Check sheet for the modelled part. Datum: model origin and axes. Units: mm. A direction names the side the tool comes from. Coordinates: 2 decimals unless noted, no trailing zeros. Write each loop counter-clockwise with the first axis right and the second up, starting at its lowest first coordinate (ties: lowest second). Pieces come first, ordered by that corner, then holes. Notation, with made-up numbers: (-23, 42.5) -> (-5, 42.5) arc R13 ccw to (-5, 58.5) -> close; hole circle Ø9 at (23, 33). An arc over 180 degrees is marked (long way). One line per item, written item: value. Start each with the question number.
1) Sectioned sample at B-B on x = 26. Enter the section's corners in (y, z).
2) Draft check along Y on faces 3 (the flat face through (7, -30, 19)), 4 (the flat face through (7, 0, 0)), 5 (the flat face through (7, 0, 2)). Enter one of: +Y half, -Y half, draft (parallel to the pull), parting line (faces both ways), or undercut.
3) Sectioned sample at A-A on z = 6. Enter the section's corners in (x, y), plus the area to 3 significant figures.
4) Sectioned sample at D-D on y = -6. Enter the section's corners in (x, z).
5) Gauge pin test, flat ends, axial feed: P1, Ø3, axis at x = 40.5, y = 5.5, coming from the +Z side; P2, Ø10, axis at x = 42, y = -14.5, coming from the +Z side. Record the tip position at first contact, or that the pin passes through.
6) Set-up check for faces 1 (the flat face through (-48, 0, 19)), 2 (the flat face through (39, 21.5, 7)): record each of +Z, -Z, +X, -X, +Y, -Y from which the full face is reachable in a straight line by a thin tool's end or side.
7) Scan lines: line 1 along X through (y, z) = (-12, 11); line 2 along X through (y, z) = (24.5, 24); line 3 along Y through (x, z) = (-6.5, 19). Record each from-to range of solid material in increasing order. Write a range as [from, to].
8) Sectioned sample at C-C on z = 21. Enter the section's corners in (x, y).
```python
from build123d import *

# Parameters (mm, degrees)
SKETCH004_W     = 112
SKETCH004_H     = 60
PAD004_DEPTH    = 38
SKETCH006_W     = 108
SKETCH006_H     = 56
POCKET002_DEPTH = 36
PAD005_DEPTH    = 10


with BuildPart() as part:
    # Sketch004 → Pad004 (new body)
    with BuildSketch(Plane.XY):
        with Locations((8, 0)):
            Rectangle(SKETCH004_W, SKETCH004_H)
    extrude(amount=PAD004_DEPTH)

    # Sketch006 (on Face6 of Pad004) → Pocket002 (cut)
    with BuildSketch(Plane.XY.offset(38)):
        with Locations((8, 0)):
            Rectangle(SKETCH006_W, SKETCH006_H)
    extrude(amount=-POCKET002_DEPTH, mode=Mode.SUBTRACT)

    # Sketch007 (on Face11 of Pocket002) → Pad005 (join)
    with BuildSketch(Plane.XY.offset(2)):
        Polygon((-36.25, 21.5), (-36.25, -21.5), (-30.25, -21.5), (-30.25, -25), (-40.25, -25), (-40.25, 25), (-30.25, 25), (-30.25, 21.5), align=None)
        Polygon((42.25, -21.5), (42.25, 21.5), (36.25, 21.5), (36.25, 25), (46.25, 25), (46.25, -25), (36.25, -25), (36.25, -21.5), align=None)
    extrude(amount=PAD005_DEPTH)


solid = part.part
```
Answers:
1. outline: (-30, 0) -> (30, 0) -> (30, 38) -> (28, 38) -> (28, 2) -> (-28, 2) -> (-28, 38) -> (-30, 38) -> close
2. face 3: -Y half
2. face 4: draft
2. face 5: undercut
3. outline: (-48, -30) -> (64, -30) -> (64, 30) -> (-48, 30) -> close; (-40.25, -25) -> (-30.25, -25) -> (-30.25, -21.5) -> (-36.25, -21.5) -> (-36.25, 21.5) -> (-30.25, 21.5) -> (-30.25, 25) -> (-40.25, 25) -> close; (36.25, -25) -> (46.25, -25) -> (46.25, 25) -> (36.25, 25) -> (36.25, 21.5) -> (42.25, 21.5) -> (42.25, -21.5) -> (36.25, -21.5) -> close; hole (-46, -28) -> (62, -28) -> (62, 28) -> (-46, 28) -> close
3. area: 1,160 mm2
4. outline: (-48, 0) -> (64, 0) -> (64, 38) -> (62, 38) -> (62, 2) -> (46.25, 2) -> (46.25, 12) -> (42.25, 12) -> (42.25, 2) -> (-36.25, 2) -> (-36.25, 12) -> (-40.25, 12) -> (-40.25, 2) -> (-46, 2) -> (-46, 38) -> (-48, 38) -> close
5. P1: stops at z = 2
5. P2: stops at z = 12
6. face 1: +Z, -Z, -X, +Y, -Y
6. face 2: +Z
7. line 1: x = [-48, -46], [-40.25, -36.25], [42.25, 46.25], [62, 64]
7. line 2: x = [-48, -46], [62, 64]
7. line 3: y = [-30, -28], [28, 30]
8. outline: (-48, -30) -> (64, -30) -> (64, 30) -> (-48, 30) -> close; hole (-46, -28) -> (62, -28) -> (62, 28) -> (-46, 28) -> close
